Build history of the part. All positions in model axes, mm. Face numbers are marked on the shaded views. A direction names the side the tool comes from. Round coordinates to 2 decimals unless told otherwise and drop trailing zeros. Write each loop counter-clockwise with the first axis right and the second up, starting at its lowest first coordinate (ties: lowest second). Pieces come first, ordered by that corner, then holes. Notation, with made-up numbers: M -4,31 L 32,31 A17 ccw 32,51 Z; hole C 59.25,86.25 d2. An arc over 180 degrees is marked long. Use a Markdown table: item, result.
from build123d import *

# Parameters (mm, degrees)
F0_W         = 11
F0_H         = 17.25
F1_DEPTH     = 8.5
F2_W         = 7.8
F2_H         = 2.55
F2_H_2       = 6
F2_W_2       = 1.6
F3_DEPTH     = 4.5
F4_W         = 5.1
F4_H         = 4
F5_DEPTH     = 6.1
F6_R         = 3.8
F7_DEPTH     = 2.5
F8_R         = 1.9
F9_DEPTH     = 1.501
F10_T1_DEPTH = 26.4746859277
F11_R        = 1
F12_R        = 0.5


# Not quite as in the source:
# - a fillet or chamfer that OpenCascade refuses, or shapes differently, is made with other operations: its cross-section is extruded or revolved along the edge and cut away or added


with BuildPart() as f1:
    # F0 (on Top) → F1 (new body)
    with BuildSketch(Plane.XY):
        Rectangle(F0_W, F0_H)
    extrude(amount=F1_DEPTH)

    # F2 (on face) → F3 (cut)
    with BuildSketch(Plane.XY.offset(8.5)):
        with Locations((0, -4.275)):
            Rectangle(F2_W, F2_H)
        Rectangle(F2_W, F2_H_2)
        with Locations((4.7, 0)):
            Rectangle(F2_W_2, F2_H_2)
        with Locations((-4.7, 0)):
            Rectangle(F2_W_2, F2_H_2)
        with Locations((0, 4.275)):
            Rectangle(F2_W, F2_H)
    extrude(amount=-F3_DEPTH, mode=Mode.SUBTRACT)

    # F4 (on face) → F5 (cut)
    with BuildSketch(Plane(origin=(0, 0, 0), x_dir=(1, 0, 0), z_dir=(0, 0, -1))):
        with Locations((0, -6.625)):
            Rectangle(F4_W, F4_H)
        with Locations((0, 6.625)):
            Rectangle(F4_W, F4_H)
    extrude(amount=-F5_DEPTH, mode=Mode.SUBTRACT)

    # F6 (on face) → F7 (cut)
    with BuildSketch(Plane.XY.offset(4)):
        Circle(F6_R)
    extrude(amount=-F7_DEPTH, mode=Mode.SUBTRACT)

    # F8 (on face) → F9 (cut, through all)
    with BuildSketch(Plane.XY.offset(1.5)):
        Circle(F8_R)
    extrude(amount=-F9_DEPTH, mode=Mode.SUBTRACT)

    # F10: fillet of radius 5 on 2 edges, made by hand

    # F10_s2 → F10_t1 (cut)
    with BuildSketch(Plane.YZ.offset(-17.9373429638)):
        with BuildLine():
            ThreePointArc((-7.9749371855, 8.5), (-4.6208352193, 7.2080992435), (-3, 4))
            Line((-3, 4), (-3, 8.5))
            Line((-3, 8.5), (-7.9749371855, 8.5))
        make_face()
        with BuildLine():
            ThreePointArc((7.9749371855, 8.5), (4.6208352193, 7.2080992435), (3, 4))
            Line((3, 4), (3, 8.5))
            Line((3, 8.5), (7.9749371855, 8.5))
        make_face()
    extrude(amount=F10_T1_DEPTH, mode=Mode.SUBTRACT)

    # F11
    f11_edges = [f1.edges().sort_by_distance(p)[0] for p in [
        (5.5, -8.625, 4.25),
        (-5.5, -8.625, 4.25),
        (5.5, 8.625, 4.25),
        (-5.5, 8.625, 4.25),
    ]]
    fillet(f11_edges, radius=F11_R)

    # F12
    f12_edges = [f1.edges().sort_by_distance(p)[0] for p in [
        (0, 8.625, 8.5),
        (0, -8.625, 8.5),
        (-5.5, 0, 4),
        (5.5, 0, 4),
        (5.5, -4.493052, 7.088381),
        (5.5, 4.493052, 7.088381),
        (5.483858, -7.803952, 8.497076),
        (5.070115, -8.446565, 8.5),
        (5.483858, 7.803952, 8.497076),
        (5.070115, 8.446565, 8.5),
        (-5.5, -4.493052, 7.088381),
        (-5.483858, -7.803951, 8.497076),
        (-5.5, 4.493052, 7.088381),
        (-5.483858, 7.803952, 8.497076),
        (-5.070115, -8.446565, 8.5),
        (-5.070115, 8.446565, 8.5),
    ]]
    fillet(f12_edges, radius=F12_R)


solid = f1.part
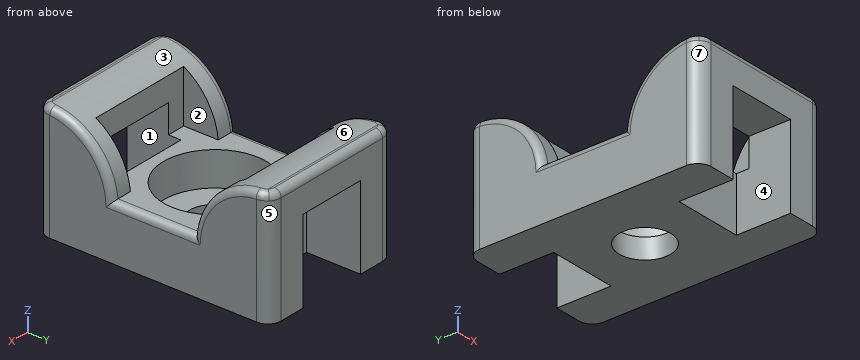
Q1. Cut at D-D on y = -2.75. Give the cut face in (x, z).
Response values:
| item | result |
|---|---|
| outline | M -5.5,0 L 5.5,0 L 5.5,3.5 A0.5 ccw 5,4 L 2.62,4 L 2.62,1.5 L -2.62,1.5 L -2.62,4 L -5,4 A0.5 ccw -5.5,3.5 Z |
Q2. Cut at B-B on y = -1. Give the cut face in (x, z), and give its area (3 significant figures).
Response values:
| item | result |
|---|---|
| outline | M -5.5,0 L -1.62,0 L -1.62,1.5 L -3.67,1.5 L -3.67,4 L -5,4 A0.5 ccw -5.5,3.5 Z; M 1.62,0 L 5.5,0 L 5.5,3.5 A0.5 ccw 5,4 L 3.67,4 L 3.67,1.5 L 1.62,1.5 Z |
| area | 20.7 mm2 |
Q3. Two-plate mould, pull along Y, no slides. Class the marked faces 4, 5, 6 and 7: +Y half, -Y half, draft (parallel to the pull), parting line (faces both ways), or undercut.
Response values:
| item | result |
|---|---|
| face 4 | draft |
| face 5 | +Y half |
| face 6 | undercut |
| face 7 | -Y half |
Q4. Drop flat-ended pins along their axis: P1, Ø3, axis at x = 0, y = 0, coming from the -Z side; P2, Ø2.5, axis at x = -1, y = 8, coming from the -Z side; P3, Ø1.3, axis at y = -4, z = 7, coming from the -X side; P4, Ø3, axis at x = 4, y = -2, coming from the +Z side. Give the stop position or say it passes through.
Response values:
| item | result |
|---|---|
| P1 | passes through |
| P2 | stops at z = 6.1 |
| P3 | stops at x = -5.48 |
| P4 | stops at z = 5.73 |
Q5. Cut at A-A on x = 0. Give the cut face in (y, z) (3 decimals).
Response values:
| item | result |
|---|---|
| outline | M -8.625,6.1 L -5.55,6.1 L -5.55,7.873 A5 ccw -7.975,8.5 L -8.125,8.5 A0.5 ccw -8.625,8 Z; M -4.625,0 L -1.9,0 L -1.9,1.5 L -3.8,1.5 L -3.8,4 L -4.625,4 Z; M 1.9,0 L 4.625,0 L 4.625,4 L 3.8,4 L 3.8,1.5 L 1.9,1.5 Z; M 5.55,6.1 L 8.625,6.1 L 8.625,8 A0.5 ccw 8.125,8.5 L 7.975,8.5 A5 ccw 5.55,7.873 Z |
Q6. Drill centre lines: L1, parallel to X at y = 0, z = 3; L2, parallel to Y at x = 0, z = 3.3 (3 decimals); L3, parallel to Y at x = 0, z = 0.4 (3 decimals). Where is each one in solid material? Low to high.
Response values:
| item | result |
|---|---|
| L1 | x = -5.5 to -3.8, 3.8 to 5.5 |
| L2 | y = -4.625 to -3.8, 3.8 to 4.625 |
| L3 | y = -4.625 to -1.9, 1.9 to 4.625 |
Q7. Which spindle directions (+Z, -Z, +X, -X, +Y, -Y) get a long thin tool onto all of the face, cutting with end or side? Do the marked faces 1, 2 and 3. Say none if no direction does.
Response values:
| item | result |
|---|---|
| face 1 | -Z, -Y |
| face 2 | +Z |
| face 3 | +Z, +X, -X |
Q8. Cut at C-C on z = 5. Count the separate pieces of the cut face and the enclosed holes in it, and give its area (3 significant figures).
Response values:
| item | result |
|---|---|
| separate pieces | 4 |
| enclosed holes | 0 |
| area | 50.2 mm2 |
